Verification items for the finished model (mm, model axes). Face numbers are marked on the shaded views. Round coordinates to 2 decimals unless told otherwise and drop trailing zeros. Loops run counter-clockwise (first coordinate to the right, second up) from the corner with the lowest first, then second, coordinate; pieces in that order, holes last. Notation, with made-up numbers: M -28,88.5 L 5,88.5 A25 ccw 5,115.5 Z; hole C -31.75,58.25 d4. An arc over 180 degrees is marked long. One line per item, written item: value.
from build123d import *

# Parameters (mm, degrees)
FILLET1_R     = 1
CHAMFER1_SIZE = 1
FILLET2_R     = 1


with BuildPart() as part:
    # Sketch1 → Revolve1 (revolve)
    with BuildSketch(Plane(origin=(0, 0, 0), x_dir=(1, 0, 0), z_dir=(0, 1, 0))):
        Polygon((34.068196428, 24.638), (34.068196428, 12.7), (35.8775, 0), (39.751, 0), (39.751, 12.7), (36.910196428, 12.7), (36.910196428, 29.718), (31.068196428, 29.718), (31.068196428, 24.638), align=None)
    revolve(axis=Axis((0, 0, 0), (0, 0, -1)))

    # Fillet1
    fillet1_edges = [part.edges().sort_by_distance(p)[0] for p in [
        (-36.910196428, 0, -12.7),
    ]]
    fillet(fillet1_edges, radius=FILLET1_R)

    # Chamfer1
    chamfer1_edges = [part.edges().sort_by_distance(p)[0] for p in [
        (-31.068196428, 0, -29.718),
    ]]
    chamfer(chamfer1_edges, length=CHAMFER1_SIZE)

    # Fillet2
    fillet2_edges = [part.edges().sort_by_distance(p)[0] for p in [
        (-34.068196428, 0, -24.638),
    ]]
    fillet(fillet2_edges, radius=FILLET2_R)


solid = part.part
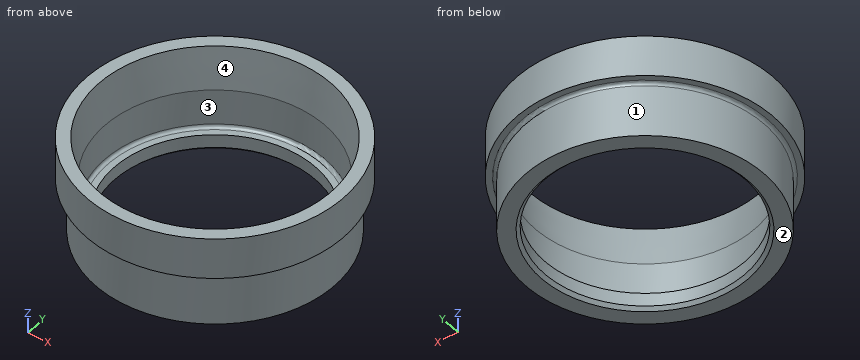
(1) Sectioned sample at C-C on z = -18.5. Enter the section's corners in (x, y), and give its area (3 significant figures).
Completed:
outline: C 0,0 d73.82; hole C 0,0 d68.14
area: 634 mm^2
(2) Mould release check, pull along X, two halves, no side actions. Record for the marked faces 1, 2, 3 and 4: +X half, -X half, draft (parallel to the pull), parting line (faces both ways), or undercut.
Completed:
face 1: parting line
face 2: draft
face 3: undercut
face 4: undercut
(3) Depth check by flat-ended pin: pin 1 Ø12 at (x, z) = (4.5, -3.5) entering from -Y; pin 2 Ø5 at (y, z) = (-27, -19) entering from -X; pin 3 Ø6 at (x, z) = (7, -3) entering from +Y; pin 4 Ø6 at (x, y) = (-2, 26) entering from -Z. Enter the tip coordinate at first touch or a pass-through.
Completed:
pin 1: stops at y = -39.75
pin 2: stops at x = -27.61
pin 3: stops at y = 39.55
pin 4: passes through
(4) Thickness scan on L1, parallel to Y at x = 0, z = -19.5; L2, parallel to Y at x = 0, z = -27.55. Record the ranges inside material, lowest first. Write a range as from..to.
Completed:
L1: y = -36.91..-34.07, 34.07..36.91
L2: y = -36.91..-31.07, 31.07..36.91
(5) Sectioned sample at A-A on y = 0. Enter the section's corners in (x, z), and give its area (3 significant figures).
Completed:
outline: M -39.75,-12.7 L -37.91,-12.7 A1 cw -36.91,-13.7 L -36.91,-29.72 L -32.07,-29.72 L -31.07,-28.72 L -31.07,-24.64 L -33.07,-24.64 A1 cw -34.07,-23.64 L -34.07,-12.7 L -35.88,0 L -39.75,0 Z; M 31.07,-28.72 L 32.07,-29.72 L 36.91,-29.72 L 36.91,-13.7 A1 cw 37.91,-12.7 L 39.75,-12.7 L 39.75,0 L 35.88,0 L 34.07,-12.7 L 34.07,-23.64 A1 cw 33.07,-24.64 L 31.07,-24.64 Z
area: 248 mm^2
